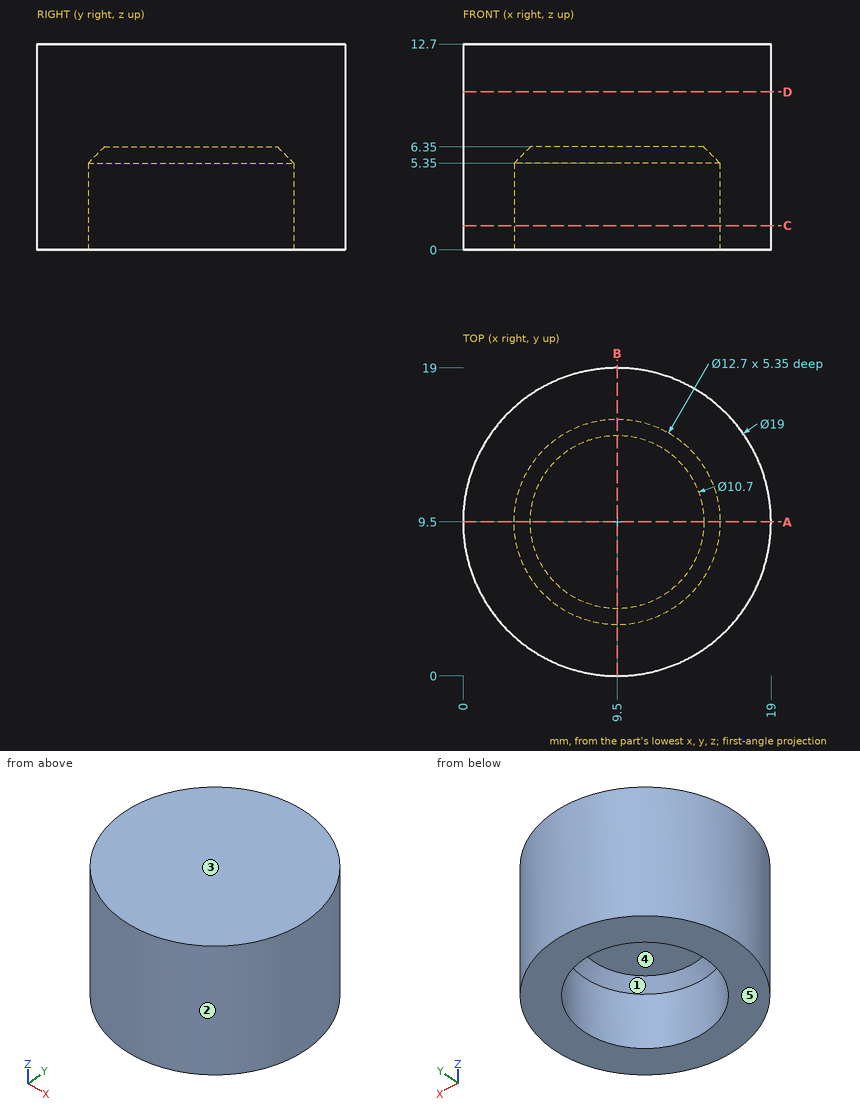
Here's the drawing with two shaded views (mm, measured from the low corner). I have some questions. A direction names the side the tool comes from. Give positions to 0.01 mm unless a question says otherwise; leave off trailing zeros. Loops run counter-clockwise (first coordinate to the right, second up) from the corner with the lowest first, then second, coordinate; pieces in that order, holes last. Notation, with made-up numbers: M 16.25,23.5 L 74.25,23.5 A22 cw 74.25,40.5 Z; hole C 42,2.5 d7. An arc over 180 degrees is marked long. Answer in a Markdown table with one row per item.
1. Suppose I cut it at C-C on z = 1.5. Write out the boundary of the cut face in (x, y).
Taken from the geometry:
| item | result |
|---|---|
| outline | C 9.5,9.5 d19; hole C 9.5,9.5 d12.7 |
2. Thinking about a two-plate mould opening in X: for the marked faces 1, 2 and 3, which applies, released by +X, released by -X, zero draft, split by the parting line, or undercut?
Taken from the geometry:
| item | result |
|---|---|
| face 1 | undercut |
| face 2 | split by the parting line |
| face 3 | zero draft |
3. For pin 1 Ø1.5 at (x, z) = (11, 10.5) entering from +Y; pin 2 Ø2 at (x, y) = (8.5, 14.5) entering from -Z; pin 3 Ø3 at (x, z) = (6.5, 2.5) entering from -Y, each with a flat end and sliding along its axis, tell me the tip position at first contact or that it passes through.
Taken from the geometry:
| item | result |
|---|---|
| pin 1 | stops at y = 18.97 |
| pin 2 | stops at z = 5.6 |
| pin 3 | stops at y = 0.12 |
4. Which directions (+Z, -Z, +X, -X, +Y, -Y) give clear straight access to the entire face, cutting with the end or side of a thin tool? Please do the marked faces 4 and 5.
Taken from the geometry:
| item | result |
|---|---|
| face 4 | -Z |
| face 5 | -Z, +X, -X, +Y, -Y |
5. Suppose I cut it at A-A on y = 9.5. Write out the boundary of the cut face in (x, z).
Taken from the geometry:
| item | result |
|---|---|
| outline | M 0,0 L 3.15,0 L 3.15,5.35 L 4.15,6.35 L 14.85,6.35 L 15.85,5.35 L 15.85,0 L 19,0 L 19,12.7 L 0,12.7 Z |
6. Suppose I cut it at D-D on z = 9.75. Write out the boundary of the cut face in (x, y).
Taken from the geometry:
| item | result |
|---|---|
| outline | C 9.5,9.5 d19 |
7. If I drill on line 1 along Y through (x, z) = (9.5, 2.8); line 2 along Z through (x, y) = (7, 13); line 3 along Y through (x, z) = (13.75, 5), over which ranges is the centre line in solid material (lowest first)?
Taken from the geometry:
| item | result |
|---|---|
| line 1 | y = 0 to 3.15, 15.85 to 19 |
| line 2 | z = 6.35 to 12.7 |
| line 3 | y = 1 to 4.78, 14.22 to 18 |
